```python
from build123d import *

# Parameters (mm, degrees)
BOSS_EXTRUDE1_DEPTH = 3
CUT_EXTRUDE1_DEPTH  = 3
SKETCH4_W           = 9.1
SKETCH4_H           = 1.6
SKETCH4_W_2         = 1.6
SKETCH4_H_2         = 9.1
CUT_EXTRUDE2_DEPTH  = 1.5
SKETCH7_R           = 1.5
CUT_EXTRUDE4_DEPTH  = 3


with BuildPart() as part:
    # Sketch2 → Boss-Extrude1 (new body)
    with BuildSketch(Plane(origin=(0, 0, 0), x_dir=(1, 0, 0), z_dir=(0, 1, 0))):
        Polygon((0, 24.84662833), (-12.423314165, 21.517811332), (-21.517811332, 12.423314165), (-24.84662833, 0), (-21.517811332, -12.423314165), (-12.423314165, -21.517811332), (0, -24.84662833), (12.423314165, -21.517811332), (21.517811332, -12.423314165), (24.84662833, 0), (21.517811332, 12.423314165), (12.423314165, 21.517811332), align=None)
    extrude(amount=BOSS_EXTRUDE1_DEPTH)

    # Sketch3 → Cut-Extrude1 (cut)
    with BuildSketch(Plane(origin=(0, 3, 0), x_dir=(1, 0, 0), z_dir=(0, 1, 0))):
        Polygon((-3.35, 23.948998535), (0, 24.84662833), (3.35, 23.948998535), (3.35, 17.448998535), (-3.35, 17.448998535), align=None)
        Polygon((5.823314165, 16.786276002), (9.073314165, 22.415441127), (12.423314165, 21.517811332), (14.87568437, 19.065441127), (11.62568437, 13.436276002), align=None)
        Polygon((13.436276002, 11.62568437), (19.065441127, 14.87568437), (21.517811332, 12.423314165), (22.415441127, 9.073314165), (16.786276002, 5.823314165), align=None)
        Polygon((17.448998535, 3.35), (23.948998535, 3.35), (24.84662833, 0), (23.948998535, -3.35), (17.448998535, -3.35), align=None)
        Polygon((16.786276002, -5.823314165), (22.415441127, -9.073314165), (21.517811332, -12.423314165), (19.065441127, -14.87568437), (13.436276002, -11.62568437), align=None)
        Polygon((11.62568437, -13.436276002), (14.87568437, -19.065441127), (12.423314165, -21.517811332), (9.073314165, -22.415441127), (5.823314165, -16.786276002), align=None)
        Polygon((3.35, -17.448998535), (3.35, -23.948998535), (0, -24.84662833), (-3.35, -23.948998535), (-3.35, -17.448998535), align=None)
        Polygon((-5.823314165, -16.786276002), (-9.073314165, -22.415441127), (-12.423314165, -21.517811332), (-14.87568437, -19.065441127), (-11.62568437, -13.436276002), align=None)
        Polygon((-13.436276002, -11.62568437), (-19.065441127, -14.87568437), (-21.517811332, -12.423314165), (-22.415441127, -9.073314165), (-16.786276002, -5.823314165), align=None)
        Polygon((-17.448998535, -3.35), (-23.948998535, -3.35), (-24.84662833, 0), (-23.948998535, 3.35), (-17.448998535, 3.35), align=None)
        Polygon((-16.786276002, 5.823314165), (-22.415441127, 9.073314165), (-21.517811332, 12.423314165), (-19.065441127, 14.87568437), (-13.436276002, 11.62568437), align=None)
        Polygon((-11.62568437, 13.436276002), (-14.87568437, 19.065441127), (-12.423314165, 21.517811332), (-9.073314165, 22.415441127), (-5.823314165, 16.786276002), align=None)
    extrude(amount=-CUT_EXTRUDE1_DEPTH, mode=Mode.SUBTRACT)

    # Sketch4 → Cut-Extrude2 (cut)
    with BuildSketch(Plane(origin=(0, 0, 0), x_dir=(-1, 0, 0), z_dir=(0, -1, 0))):
        with Locations((0, -21.648998535)):
            Rectangle(SKETCH4_W, SKETCH4_H)
        Polygon((-6.48408368, -20.330762375), (-7.28408368, -21.716403021), (-15.164914855, -17.166403021), (-14.364914855, -15.780762375), align=None)
        Polygon((-15.780762375, -14.364914855), (-17.166403021, -15.164914855), (-21.716403021, -7.28408368), (-20.330762375, -6.48408368), align=None)
        with Locations((-21.648998535, 0)):
            Rectangle(SKETCH4_W_2, SKETCH4_H_2)
        Polygon((-20.330762375, 6.48408368), (-21.716403021, 7.28408368), (-17.166403021, 15.164914855), (-15.780762375, 14.364914855), align=None)
        Polygon((-14.364914855, 15.780762375), (-15.164914855, 17.166403021), (-7.28408368, 21.716403021), (-6.48408368, 20.330762375), align=None)
        with Locations((0, 21.648998535)):
            Rectangle(SKETCH4_W, SKETCH4_H)
        Polygon((6.48408368, 20.330762375), (7.28408368, 21.716403021), (15.164914855, 17.166403021), (14.364914855, 15.780762375), align=None)
        Polygon((15.780762375, 14.364914855), (17.166403021, 15.164914855), (21.716403021, 7.28408368), (20.330762375, 6.48408368), align=None)
        with Locations((21.648998535, 0)):
            Rectangle(SKETCH4_W_2, SKETCH4_H_2)
        Polygon((20.330762375, -6.48408368), (21.716403021, -7.28408368), (17.166403021, -15.164914855), (15.780762375, -14.364914855), align=None)
        Polygon((14.364914855, -15.780762375), (15.164914855, -17.166403021), (7.28408368, -21.716403021), (6.48408368, -20.330762375), align=None)
    extrude(amount=-CUT_EXTRUDE2_DEPTH, mode=Mode.SUBTRACT)

    # Sketch7 → Cut-Extrude4 (cut)
    with BuildSketch(Plane.XZ):
        with Locations(Location((0, 6.35, 0), (0, 0, 270))):
            Circle(SKETCH7_R)
        with Locations(Location((6.35, 0, 0), (0, 0, 270))):
            Circle(SKETCH7_R)
        with Locations(Location((0, -6.35, 0), (0, 0, 270))):
            Circle(SKETCH7_R)
        with Locations(Location((-6.35, 0, 0), (0, 0, 270))):
            Circle(SKETCH7_R)
    extrude(amount=-CUT_EXTRUDE4_DEPTH, mode=Mode.SUBTRACT)


solid = part.part
```
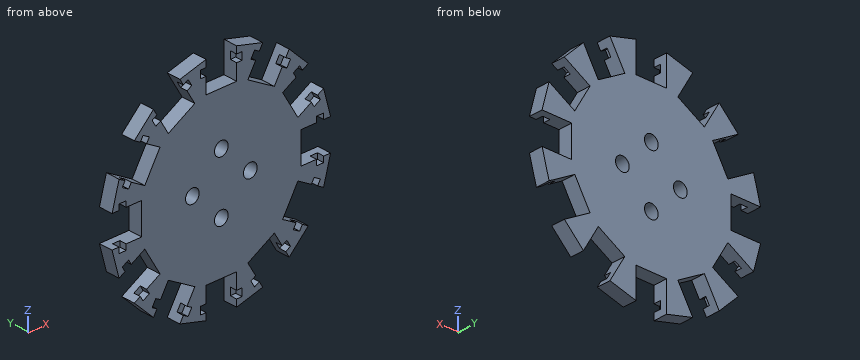
Verification items for the finished model (mm, model axes). Round coordinates to 2 decimals unless told otherwise and drop trailing zeros. Loops run counter-clockwise (first coordinate to the right, second up) from the corner with the lowest first, then second, coordinate; pieces in that order, holes last. Notation, with made-up numbers: (85, -16.75) -> (102, -16.75) arc R21 cw to (102, 5.25) -> close; hole circle Ø5 at (50, -19). An arc over 180 degrees is marked (long way). Answer as a JSON object with one key per item and string values.
Q1. Section check D-D (z = -11). Record the boundary of the cut face in (x, y), then the cut area to 3 significant figures.
Data:
{"outline": "(-13.8, 0) -> (13.8, 0) -> (13.8, 3) -> (-13.8, 3) -> close", "area": "82.8 mm2"}
Q2. Go/stop test with flat-tipped pins: P1, Ø1.2, axis at y = 0.5, z = -21.5, coming from the -X side; P2, Ø1.2, axis at y = 0.5, z = 22, coming from the -X side; P3, Ø1, axis at y = 1, z = 14, coming from the +X side. Record where each tip stops, or that it passes through.
Data:
{"P1": "stops at x = -8.89", "P2": "stops at x = -9.07", "P3": "stops at x = 18.41"}
Q3. Section check B-B (x = 0). Record the boundary of the cut face in (y, z), then the cut area to 3 significant figures.
Data:
{"outline": "(0, -17.45) -> (3, -17.45) -> (3, -7.85) -> (0, -7.85) -> close; (0, -4.85) -> (3, -4.85) -> (3, 4.85) -> (0, 4.85) -> close; (0, 7.85) -> (3, 7.85) -> (3, 17.45) -> (0, 17.45) -> close", "area": "86.7 mm2"}
Q4. Scan lines: line 1 (X direction, y = 1.2, z = 0); line 2 (Z direction, x = -18, y = 1.55); line 3 (X direction, y = 2.55, z = 1). Record each from-to range of solid material in increasing order. Write a range as from..to.
Data:
{"line 1": "x = -17.45..-7.85, -4.85..4.85, 7.85..17.45", "line 2": "z = -15.94..-14.26, -6.52..-3.35, 3.35..6.52, 14.26..15.94", "line 3": "x = -17.45..-7.47, -5.23..5.23, 7.47..17.45"}
Q5. Section check A-A (z = 0). Record the boundary of the cut face in (x, y), then the cut area to 3 significant figures.
Data:
{"outline": "(-17.45, 0) -> (-7.85, 0) -> (-7.85, 3) -> (-17.45, 3) -> close; (-4.85, 0) -> (4.85, 0) -> (4.85, 3) -> (-4.85, 3) -> close; (7.85, 0) -> (17.45, 0) -> (17.45, 3) -> (7.85, 3) -> close", "area": "86.7 mm2"}
Q6. Section check C-C (y = 0.7). State how many separate pieces and enclosed holes the cut face has, then the cut area to 3 significant figures.
Data:
{"separate pieces": "1", "enclosed holes": "4", "area": "1,220 mm2"}
